Input: part model. Units: mm. Frame: model coordinates. Give positions to 0.01 mm unless a question says otherwise; leave off trailing zeros. Order: outer loops, then holes, each group sorted by start corner. A loop starts at its lowest first (then second) coordinate and runs counter-clockwise, first axis right, second up. Notation, with made-up numbers: M -29,-15 L 17,-15 A12 ccw 17,2 Z; hole C 34.5,28.5 d4. An arc over 180 degrees is marked long. Use a Markdown table: item, result.
from build123d import *

# Parameters (mm, degrees)
F0_W     = 10
F0_H     = 12.9
F1_DEPTH = 9.6
F3_DEPTH = 10.001
F4_R     = 2


with BuildPart() as f1:
    # F0 (on Top) → F1 (new body)
    with BuildSketch(Plane.XY):
        Rectangle(F0_W, F0_H)
    extrude(amount=F1_DEPTH)

    # F2 (on face) → F3 (cut, through all)
    with BuildSketch(Plane(origin=(-5, 0, 0), x_dir=(0, -1, 0), z_dir=(-1, 0, 0))):
        with BuildLine():
            Line((-4.8, 6.15), (0, 6.15))
            Line((0, 6.15), (4.8, 6.15))
            ThreePointArc((4.8, 6.15), (4.419219, 8.023634), (3.337289, 9.6))
            Line((3.337289, 9.6), (-3.337289, 9.6))
            ThreePointArc((-3.337289, 9.6), (-4.419219, 8.023634), (-4.8, 6.15))
        make_face()
        with BuildLine():
            ThreePointArc((-4.8, 6.15), (-3.394113, 2.755887), (0, 1.35))
            Line((0, 1.35), (0, 6.15))
            Line((0, 6.15), (-4.8, 6.15))
        make_face()
        with BuildLine():
            Line((0, 6.15), (0, 1.35))
            ThreePointArc((0, 1.35), (3.394113, 2.755887), (4.8, 6.15))
            Line((4.8, 6.15), (0, 6.15))
        make_face()
    extrude(amount=-F3_DEPTH, mode=Mode.SUBTRACT)

    # F4
    f4_edges = [f1.edges().sort_by_distance(p)[0] for p in [
        (0, -6.45, 0),
        (0, 6.45, 0),
    ]]
    fillet(f4_edges, radius=F4_R)


solid = f1.part
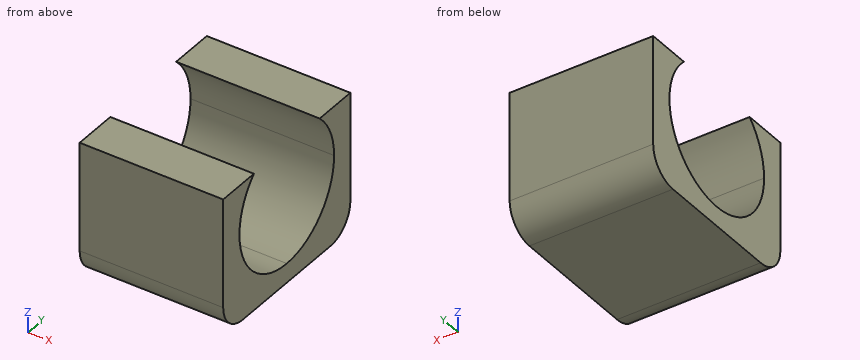
1) Cut plane A-A on x = 4. Return loops of the section in (y, z), and give its area (3 significant figures).
Response values:
| item | result |
|---|---|
| outline | M -6.45,2 A2 ccw -4.45,0 L 4.45,0 A2 ccw 6.45,2 L 6.45,9.6 L 3.34,9.6 A4.8 cw 4.8,6.15 A4.8 cw 0,1.35 A4.8 cw -4.8,6.15 A4.8 cw -3.34,9.6 L -6.45,9.6 Z |
| area | 55.9 mm² |
2) Cut plane C-C on y = -3.5. Return loops of the section in (x, z).
Response values:
| item | result |
|---|---|
| outline | M -5,0 L 5,0 L 5,2.87 L -5,2.87 Z; M -5,9.43 L 5,9.43 L 5,9.6 L -5,9.6 Z |
3) Cut plane D-D on y = 2.75. Return loops of the section in (x, z).
Response values:
| item | result |
|---|---|
| outline | M -5,0 L 5,0 L 5,2.22 L -5,2.22 Z |
4) Material intervals for line 1 (Y direction, x = 3, z = 4); line 2 (Y direction, x = 4.75, z = 9); line 3 (Z direction, x = -1.75, y = -3), sorted ascending. Write a range as from..to.
Response values:
| item | result |
|---|---|
| line 1 | y = -6.45..-4.29, 4.29..6.45 |
| line 2 | y = -6.45..-3.86, 3.86..6.45 |
| line 3 | z = 0..2.4 |
5) Cut plane B-B on z = 3.75. Return loops of the section in (x, y).
Response values:
| item | result |
|---|---|
| outline | M -5,-6.45 L 5,-6.45 L 5,-4.16 L -5,-4.16 Z; M -5,4.16 L 5,4.16 L 5,6.45 L -5,6.45 Z |
